Autodesk Inventor part; units mm, degrees
ref_plane "YZ Plane" through (0, 0, 0) normal (1, 0, 0) x (0, 1, 0)
ref_plane "XZ Plane" through (0, 0, 0) normal (0, 1, 0) x (-1, 0, 0)
ref_plane "XY Plane" through (0, 0, 0) normal (0, 0, 1) x (1, 0, 0)
sketch "スケッチ1" plane through (0, 0, 0) normal (0, 0, 1) x (1, 0, 0)
  circle A0 centre (0, 0) radius 48.5
  circle A1 centre (0, 0) radius 46.0893
  line L0 (-50, 50) -> (50, 50)
  line L1 (50, 50) -> (50, -50)
  line L2 (50, -50) -> (-50, -50)
  line L3 (-50, -50) -> (-50, 50)
  dimension "d0" = 97
  dimension "d3" = 50
  dimension "d4" = 50
  dimension "d5" = 50
  dimension "d6" = 50
extrude "押し出し1" add sketch "スケッチ1" along normal blind 5 contours A0 | A1 | L0 L1 L2 L3
sketch "スケッチ2" plane through (0, 0, 5) normal (0, 0, 1) x (1, 0, 0)
  circle A0 centre (0, 0) radius 46
  line L0 (0, 0) -> (0, 64.6511)
  line L1 (0, 0) -> (-25.9524, 62.6547)
  line L2 (-50, 50) -> (-50, -50)
  point P0 (-17.6034, 42.4985)
  point P1 (-42.4985, 17.6034)
  point P2 (-42.4985, -17.6034)
  point P3 (-17.6034, -42.4985)
  point P4 (17.6034, -42.4985)
  point P5 (42.4985, -17.6034)
  point P6 (42.4985, 17.6034)
  point P7 (17.6034, 42.4985)
  dimension "d7" = 92
  dimension "d8" = 22.5
  dimension "d11" = 360
  dimension "d76" = 50
hole "穴1" at (-17.6034, 42.4985, 5) at (-42.4985, 17.6034, 5) at (-42.4985, -17.6034, 5) at (-17.6034, -42.4985, 5) at (17.6034, -42.4985, 5) at (42.4985, -17.6034, 5) at (42.4985, 17.6034, 5) at (17.6034, 42.4985, 5) direction (0, 0, -1) diameter 2.459 end through all
sketch "スケッチ3" plane through (0, 0, 5) normal (0, 0, 1) x (1, 0, 0)
  circle A0 centre (0, 0) radius 30
  dimension "d20" = 60
extrude "押し出し2" cut sketch "スケッチ3" against normal blind 5
sketch "スケッチ4" plane through (50, -50, 0) normal (1, 0, 0) x (0, 0, -1)
  line L0 (-5, 100) -> (-5, 0)
  line L1 (-5, 100) -> (0, 100)
  line L2 (0, 100) -> (0, 0)
  line L3 (0, 0) -> (-5, 0)
  line L4 (-5, 0) -> (-5, 100)
  point P0 (0, 50)
extrude "押し出し3" add sketch "スケッチ4" along normal blind 40
sketch "スケッチ5" plane through (0, 0, 5) normal (0, 0, 1) x (1, 0, 0)
  line L0 (-50, 50) -> (90, 50)
  line L1 (85, 50) -> (90, 50)
  line L2 (90, 50) -> (90, -50)
  line L3 (90, -50) -> (85, -50)
  line L4 (85, -50) -> (85, 50)
  line L5 (-50, -50) -> (90, -50)
  line L6 (90, 50) -> (90, -50)
  point P0 (0, 0)
  point P1 (90, 50)
  point P2 (90, 0)
  dimension "d25" = 0
  dimension "d26" = 5
  dimension "d27" = 100
  dimension "d70" = 0
extrude "押し出し4" add sketch "スケッチ5" along normal blind 100
sketch "スケッチ6" plane through (90, -50, 0) normal (1, 0, 0) x (0, 0, -1)
  circle A0 centre (-55, 50) radius 46
  line L0 (0, 0) -> (-105, 0)
  line L1 (0, 0) -> (0, 100)
  line L2 (-55, 50) -> (41.9537, 50)
  line L3 (-55, 50) -> (-55, 131.7305)
  line L4 (-55, 50) -> (-80.0101, 110.3797)
  circle A1 centre (-55, 50) radius 12.5
  line L5 (-55, 50) -> (-63.1841, 64.1753)
  point P0 (0, 50)
  point P1 (-72.6034, 92.4985)
  point P2 (-97.4985, 67.6034)
  point P3 (-97.4985, 32.3966)
  point P4 (-72.6034, 7.5015)
  point P5 (-37.3966, 7.5015)
  point P6 (-12.5015, 32.3966)
  point P7 (-12.5015, 67.6034)
  point P8 (-37.3966, 92.4985)
  point P9 (-61.25, 60.8253)
  point P10 (-67.5, 50)
  point P11 (-61.25, 39.1747)
  point P12 (-48.75, 39.1747)
  point P13 (-42.5, 50)
  point P14 (-48.75, 60.8253)
  dimension "d32" = 92
  dimension "d34" = 25
  dimension "d30" = 50
  dimension "d31" = 55
  dimension "d33" = 22.5
  dimension "d35" = 30
  dimension "d38" = 360
  dimension "d42" = 360
hole "穴2" at (90, 42.4985, 72.6034) at (90, 17.6034, 97.4985) at (90, -17.6034, 97.4985) at (90, -42.4985, 72.6034) at (90, -42.4985, 37.3966) at (90, -17.6034, 12.5015) at (90, 17.6034, 12.5015) at (90, 42.4985, 37.3966) at (90, 10.8253, 61.25) at (90, 0, 67.5) at (90, -10.8253, 61.25) at (90, -10.8253, 48.75) at (90, 0, 42.5) at (90, 10.8253, 48.75) direction (-1, 0, 0) diameter 2.459 end through all
sketch "スケッチ7" plane through (90, -50, 0) normal (1, 0, 0) x (0, 0, -1)
  line L0 (-55, 50) -> (26.223, 50)
  circle A0 centre (-55, 50) radius 10.2
  line L1 (0, 0) -> (0, 100)
  line L2 (0, 0) -> (-105, 0)
  line L3 (-55, 50) -> (-55, 82.0983)
  point P0 (0, 50)
  point P1 (-55, 60.2)
  point P2 (-63.8335, 44.9)
  point P3 (-46.1665, 44.9)
  dimension "d53" = 20.4
  dimension "d51" = 55
  dimension "d52" = 50
  dimension "d56" = 360
hole "穴3" at (90, 10.2, 55) at (90, -5.1, 63.8335) at (90, -5.1, 46.1665) direction (-1, 0, 0) diameter 4 end through all
sketch "スケッチ8" plane through (90, -50, 0) normal (1, 0, 0) x (0, 0, -1)
  circle A0 centre (-55, 50) radius 6.5
  line L0 (0, 0) -> (0, 100)
  line L1 (0, 0) -> (-105, 0)
  point P0 (0, 50)
  dimension "d65" = 13
  dimension "d66" = 55
  dimension "d67" = 50
extrude "押し出し5" cut sketch "スケッチ8" against normal through all
sketch "スケッチ9" plane through (0, 0, 105) normal (0, 0, 1) x (1, 0, 0)
  line L0 (-50, 50) -> (85, 50)
  line L1 (-50, -50) -> (90, -50)
  line L2 (85, 50) -> (90, 50)
  line L3 (90, 50) -> (90, -50)
  line L4 (90, -50) -> (85, -50)
  line L5 (85, -50) -> (85, 50)
  point P0 (0, 0)
extrude "押し出し6" add sketch "スケッチ9" along normal blind 5
sketch "スケッチ10" plane through (85, -50, 5) normal (-1, 0, 0) x (0, 0, 1)
  line L0 (105, 100) -> (105, 0)
  line L1 (-5, 0) -> (105, 0)
  line L2 (105, 100) -> (100, 100)
  line L3 (100, 100) -> (100, 0)
  line L4 (100, 0) -> (105, 0)
  line L5 (105, 0) -> (105, 100)
  point P0 (-5, 50)
  dimension "d73" = 5
extrude "押し出し7" add sketch "スケッチ10" along normal blind 135
sketch "スケッチ11" plane through (0, 0, 110) normal (0, 0, 1) x (1, 0, 0)
  circle A0 centre (0, 0) radius 46
  line L0 (0, 0) -> (0, 49.674)
  line L1 (0, 0) -> (-20.8641, 50.3704)
  point P0 (-17.6034, 42.4985)
  point P1 (-42.4985, 17.6034)
  point P2 (-42.4985, -17.6034)
  point P3 (-17.6034, -42.4985)
  point P4 (17.6034, -42.4985)
  point P5 (42.4985, -17.6034)
  point P6 (42.4985, 17.6034)
  point P7 (17.6034, 42.4985)
  dimension "d79" = 92
  dimension "d80" = 22.5
  dimension "d81" = 360
hole "穴4" at (-17.6034, 42.4985, 110) at (17.6034, 42.4985, 110) at (42.4985, 17.6034, 110) at (42.4985, -17.6034, 110) at (17.6034, -42.4985, 110) at (-17.6034, -42.4985, 110) at (-42.4985, -17.6034, 110) at (-42.4985, 17.6034, 110) direction (0, 0, -1) diameter 2.459 end through all
sketch "スケッチ12" plane through (0, 0, 110) normal (0, 0, 1) x (1, 0, 0)
  circle A0 centre (0, 0) radius 30
  circle A1 centre (0, 0) radius 30
extrude "押し出し8" cut sketch "スケッチ12" against normal blind 135
properties part number "legparts_07(three)"
The listing builds one solid part. Answer for the finished solid, in the listing's coordinates (mm). A direction names the side the tool comes from. Coordinates: 2 decimals unless noted, no trailing zeros. Loops run counter-clockwise (first coordinate to the right, second up) from the corner with the lowest first, then second, coordinate; pieces in that order, holes last. Notation, with made-up numbers: M -13,-23 L -3,-23 A27 cw -3,-4 Z; hole C 56.25,76 d3. An arc over 180 degrees is marked long. Answer as a JSON object with one key per item and string values. Group by question number.
Item 1: Section B-B (y = -26.5) is taken. Write down the section's boundary in (x, z), and give its area (3 significant figures).
Item 2: Consider L1, parallel to Z at x = -39, y = -13.5; L2, parallel to Y at x = 88, z = 55; L3, parallel to Y at x = 88.2, z = 42.5. Determine where each line is inside the solid, lowest interval first.
Item 3: Which of the six approach directions +Z, -Z, +X, -X, +Y, -Y give full straight-line access (tool end or side, diameter ignored) to faces 4 (the face through (33, 1, 105)), 5 (the face through (87.465, 12.152, 55.434))?
Item 4: Each of these flat-tipped pins is pushed along its axis until it touches: P1, Ø8, axis at y = 14, z = 47.5, coming from the -X side; P2, Ø1.5, axis at x = 42.5, y = 17.6, coming from the -Z side; P3, Ø5, axis at y = -5.1, z = 63.83, coming from the +X side. Where does it stop, or does it pass through?
Item 5: Section C-C (x = 0) is taken. Write down the section's boundary in (y, z).
Item 6: Section A-A (x = 46.5) is taken. Write down the section's boundary in (y, z), and give its area (3 significant figures).
Item 7: Determine the mould class of faces 1 (the face through (37, 1, 110)), 2 (the face through (-50, -1, 2)), 3 (the face through (87.46, -4.33, 44.32)) for opening direction Z: +Z half, -Z half, draft (parallel to the pull), parting line (faces both ways), or undercut.
Solved:
{
 "1": {"outline": "M -50,0 L -14.06,0 L -14.06,5 L -50,5 Z; M -50,105 L -14.06,105 L -14.06,110 L -50,110 Z; M 14.06,0 L 90,0 L 90,110 L 14.06,110 L 14.06,105 L 85,105 L 85,5 L 14.06,5 Z", "area": "1,620 mm2"},
 "2": {"L1": "z = 0 to 5, 105 to 110", "L2": "y = -50 to -6.5, 6.5 to 8.2, 12.2 to 50", "L3": "y = -50 to -1.23, 1.23 to 50"},
 "3": {"face 4": "-X, +Y, -Y", "face 5": "+X, -X"},
 "4": {"P1": "stops at x = 85", "P2": "passes through", "P3": "stops at x = 90"},
 "5": {"outline": "M -50,0 L -30,0 L -30,5 L -50,5 Z; M -50,105 L -30,105 L -30,110 L -50,110 Z; M 30,0 L 50,0 L 50,5 L 30,5 Z; M 30,105 L 50,105 L 50,110 L 30,110 Z"},
 "6": {"outline": "M -50,0 L 50,0 L 50,5 L -50,5 Z; M -50,105 L 50,105 L 50,110 L -50,110 Z", "area": "1,000 mm2"},
 "7": {"face 1": "+Z half", "face 2": "draft", "face 3": "undercut"}
}
